Answer from the drawing. Dimensions are ordinates in mm from the lowest x, y and z of the part. A direction names the side the tool comes from. Give positions to 0.01 mm unless a question says otherwise; leave off trailing zeros. Order: outer loops, then holes, each group sorted by start corner. A loop starts at its lowest first (then second) coordinate and runs counter-clockwise, first axis right, second up.
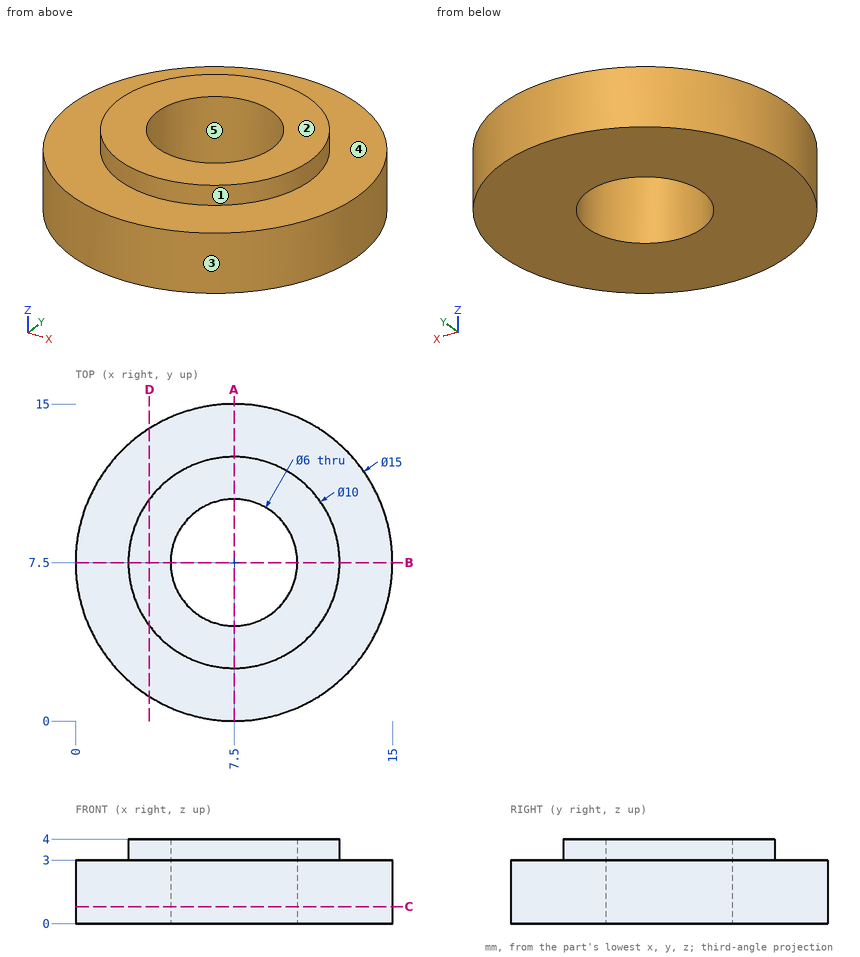
1) For a pull along X with two mould halves and no side action, classify the marked faces 3, 4 and 5 as released by +X, released by -X, zero draft, split by the parting line, or undercut.
Final values:
face 3: split by the parting line
face 4: zero draft
face 5: undercut
2) A tool of negligible diameter and unlimited length cuts with its end or side. For the marked faces 1 and 2, from which of +Z, -Z, +X, -X, +Y, -Y can it reach the whole face along a straight path? Write none if from no direction.
Final values:
face 1: +Z
face 2: +Z, +X, -X, +Y, -Y
3) The part is cut by section A-A on x = 7.5. Determine the outline of the cut face in (y, z), and give its area (3 significant figures).
Final values:
outline: (0, 0) - (4.5, 0) - (4.5, 4) - (2.5, 4) - (2.5, 3) - (0, 3) - close; (10.5, 0) - (15, 0) - (15, 3) - (12.5, 3) - (12.5, 4) - (10.5, 4) - close
area: 31.0 mm2
4) The part is cut by section C-C on z = 0.8. Determine the outline of the cut face in (x, y), and give its area (3 significant figures).
Final values:
outline: circle Ø15 at (7.5, 7.5); hole circle Ø6 at (7.5, 7.5)
area: 148 mm2
5) Consider L1, parallel to Y at x = 7.5, z = 1.6; L2, parallel to Z at x = 3.5, y = 13; L3, parallel to X at y = 9, z = 0.7. Determine where each line is inside the solid, lowest interval first.
Final values:
L1: y = 0 to 4.5, 10.5 to 15
L2: z = 0 to 3
L3: x = 0.15 to 4.9, 10.1 to 14.85
6) The part is cut by section D-D on x = 3.5. Determine the outline of the cut face in (y, z), and give its area (3 significant figures).
Final values:
outline: (1.16, 0) - (13.84, 0) - (13.84, 3) - (10.5, 3) - (10.5, 4) - (4.5, 4) - (4.5, 3) - (1.16, 3) - close
area: 44.1 mm2
7) Given pin 1 (1.5 mm diameter, centred on x = 3, z = 3, fed in from -Y); pin 2 (1 mm diameter, centred on x = 10.5, z = 3, fed in from -Y); pin 3 (2 mm diameter, centred on y = 10, z = 1, fed in from -X); pin 4 (5 mm diameter, centred on x = 7.5, y = 7.5, fed in from -Z), each flat-ended and moving along its own axis, determine where each tip first touches the part or whether it passes through.
Final values:
pin 1: stops at y = 1
pin 2: stops at y = 0.43
pin 3: stops at x = 0.15
pin 4: passes through
